from build123d import *

# Parameters (mm, degrees)
BOSS_EXTRUDE1_DEPTH = 3.175
SKETCH2_R           = 1.5875
SKETCH2_W           = 80.264
SKETCH2_H           = 12.954
CUT_EXTRUDE1_DEPTH  = 223.985606318
SKETCH7_R           = 1.5875
SKETCH7_W           = 46.99
SKETCH7_H           = 138.43
CUT_EXTRUDE4_DEPTH  = 223.985606318
CUT_EXTRUDE5_DEPTH  = 223.985606318
SKETCH9_W           = 300.072277348
SKETCH9_H           = 334.026066528
CUT_EXTRUDE6_DEPTH  = 221.482742149
SKETCH10_R          = 1.5875
CUT_EXTRUDE7_DEPTH  = 214.733203623


with BuildPart() as part:
    # Sketch1 → Boss-Extrude1 (new body)
    with BuildSketch(Plane(origin=(0, 0, 0), x_dir=(1, 0, 0), z_dir=(0, 1, 0))):
        with BuildLine():
            Line((-80, 112.5), (100, 112.5))
            Line((100, 112.5), (100, -112.5))
            Line((100, -112.5), (-80, -112.5))
            ThreePointArc((-80, -112.5), (-192.5, 0), (-80, 112.5))
        make_face()
    extrude(amount=-BOSS_EXTRUDE1_DEPTH)

    # Sketch2 → Cut-Extrude1 (cut, through all)
    with BuildSketch(Plane(origin=(0, 0, 0), x_dir=(1, 0, 0), z_dir=(0, 1, 0))):
        with Locations(Location((36.144045702, -74.2188, 0), (0, 0, 270))):
            Circle(SKETCH2_R)
        with Locations(Location((36.144045702, -67.8688, 0), (0, 0, 270))):
            Circle(SKETCH2_R)
        with Locations(Location((36.144045702, -61.5188, 0), (0, 0, 270))):
            Circle(SKETCH2_R)
        with Locations(Location((36.144045702, -55.1688, 0), (0, 0, 270))):
            Circle(SKETCH2_R)
        with Locations(Location((36.144045702, -48.8188, 0), (0, 0, 270))):
            Circle(SKETCH2_R)
        with Locations(Location((36.144045702, -42.4688, 0), (0, 0, 270))):
            Circle(SKETCH2_R)
        with Locations(Location((36.144045702, -36.1188, 0), (0, 0, 270))):
            Circle(SKETCH2_R)
        with Locations(Location((67.894045702, -74.2188, 0), (0, 0, 270))):
            Circle(SKETCH2_R)
        with Locations(Location((67.894045702, -67.8688, 0), (0, 0, 270))):
            Circle(SKETCH2_R)
        with Locations(Location((67.894045702, -61.5188, 0), (0, 0, 270))):
            Circle(SKETCH2_R)
        with Locations(Location((67.894045702, -55.1688, 0), (0, 0, 270))):
            Circle(SKETCH2_R)
        with Locations(Location((67.894045702, -48.8188, 0), (0, 0, 270))):
            Circle(SKETCH2_R)
        with Locations(Location((67.894045702, -42.4688, 0), (0, 0, 270))):
            Circle(SKETCH2_R)
        with Locations(Location((67.894045702, -36.1188, 0), (0, 0, 270))):
            Circle(SKETCH2_R)
        with Locations(Location((36.144045702, 74.2188, 0), (0, 0, 270))):
            Circle(SKETCH2_R)
        with Locations(Location((36.144045702, 67.8688, 0), (0, 0, 270))):
            Circle(SKETCH2_R)
        with Locations(Location((36.144045702, 61.5188, 0), (0, 0, 270))):
            Circle(SKETCH2_R)
        with Locations(Location((36.144045702, 55.1688, 0), (0, 0, 270))):
            Circle(SKETCH2_R)
        with Locations(Location((36.144045702, 48.8188, 0), (0, 0, 270))):
            Circle(SKETCH2_R)
        with Locations(Location((36.144045702, 42.4688, 0), (0, 0, 270))):
            Circle(SKETCH2_R)
        with Locations(Location((36.144045702, 36.1188, 0), (0, 0, 270))):
            Circle(SKETCH2_R)
        with Locations(Location((67.894045702, 74.2188, 0), (0, 0, 270))):
            Circle(SKETCH2_R)
        with Locations(Location((67.894045702, 67.8688, 0), (0, 0, 270))):
            Circle(SKETCH2_R)
        with Locations(Location((67.894045702, 61.5188, 0), (0, 0, 270))):
            Circle(SKETCH2_R)
        with Locations(Location((67.894045702, 55.1688, 0), (0, 0, 270))):
            Circle(SKETCH2_R)
        with Locations(Location((67.894045702, 48.8188, 0), (0, 0, 270))):
            Circle(SKETCH2_R)
        with Locations(Location((67.894045702, 42.4688, 0), (0, 0, 270))):
            Circle(SKETCH2_R)
        with Locations(Location((67.894045702, 36.1188, 0), (0, 0, 270))):
            Circle(SKETCH2_R)
        with Locations((52.019045702, -96.4438)):
            Rectangle(SKETCH2_W, SKETCH2_H)
        with Locations((52.019045702, 96.4438)):
            Rectangle(SKETCH2_W, SKETCH2_H)
    extrude(amount=-CUT_EXTRUDE1_DEPTH, mode=Mode.SUBTRACT)

    # Sketch7 → Cut-Extrude4 (cut, through all)
    with BuildSketch(Plane(origin=(0, 0, 0), x_dir=(1, 0, 0), z_dir=(0, 1, 0))):
        with Locations(Location((-50.166143469, 0, 0), (0, 0, 270))):
            Circle(SKETCH7_R)
        with Locations(Location((25.582761582, 0, 0), (0, 0, 270))):
            Circle(SKETCH7_R)
        with Locations(Location((87.462148806, 0, 0), (0, 0, 270))):
            Circle(SKETCH7_R)
        with Locations((-13.971143469, 0)):
            Rectangle(SKETCH7_W, SKETCH7_H)
    extrude(amount=-CUT_EXTRUDE4_DEPTH, mode=Mode.SUBTRACT)

    # Sketch8 → Cut-Extrude5 (cut, through all)
    with BuildSketch(Plane(origin=(0, 0, 0), x_dir=(1, 0, 0), z_dir=(0, 1, 0))):
        with BuildLine():
            Line((-167.0966, 25.4), (-229.776686608, 25.4))
            Line((-229.776686608, 25.4), (-229.776686608, -25.4))
            Line((-229.776686608, -25.4), (-167.0966, -25.4))
            ThreePointArc((-167.0966, -25.4), (-141.6966, 0), (-167.0966, 25.4))
        make_face()
    extrude(amount=-CUT_EXTRUDE5_DEPTH, mode=Mode.SUBTRACT)

    # Sketch9 → Cut-Extrude6 (cut, through all)
    with BuildSketch(Plane(origin=(0, 0, 0), x_dir=(1, 0, 0), z_dir=(0, 1, 0))):
        with Locations((15.89966987, 0.169857655)):
            Rectangle(SKETCH9_W, SKETCH9_H)
    extrude(amount=-CUT_EXTRUDE6_DEPTH, mode=Mode.SUBTRACT)

    # Sketch10 → Cut-Extrude7 (cut, through all)
    with BuildSketch(Plane(origin=(0, 0, 0), x_dir=(1, 0, 0), z_dir=(0, 1, 0))):
        with Locations(Location((-178.345859252, -36.864745569, 0), (0, 0, 270))):
            Circle(SKETCH10_R)
        with Locations(Location((-178.345859252, 35.885864147, 0), (0, 0, 270))):
            Circle(SKETCH10_R)
    extrude(amount=-CUT_EXTRUDE7_DEPTH, mode=Mode.SUBTRACT)


solid = part.part
Source: CAD feature listing. Evaluate the final solid. Frame: model axes, mm. A direction names the side the tool comes from. Give positions to 0.01 mm unless a question says otherwise; leave off trailing zeros. Write each loop counter-clockwise with the first axis right and the second up, starting at its lowest first coordinate (ties: lowest second). Pieces come first, ordered by that corner, then holes. Notation, with made-up numbers: M 2.5,6.25 L 32.5,6.25 A23 cw 32.5,33.25 Z; hole C 26,46.25 d10. An arc over 180 degrees is marked long. Return JSON: item names as keys, results as strings. Group by question number.
1) Set-up query: faces 5 (the face through (-179, -2, 25.4)), 6 (the face through (-137, 0, -1)). Return all of +Z, -Z, +X, -X, +Y, -Y with unobstructed straight access to the full face (end or side cutting, diameter ignored); none if empty.
2) Cut plane D-D, the plane x = -147. Output: boundary loops of the cut face in (y, z) (3 decimals).
3) Cut plane B-B, the plane y = -1. Output: boundary loops of the cut face in (x, z) (1 decimal).
4) Cut plane C-C, the plane z = 0. Output: boundary loops of the cut face in (x, y) (3 decimals), then the cut area to 3 significant figures.
5) First-contact query: pin 1 Ø10 at (x, z) = (-175.5, -72.5) entering from +Y; pin 2 Ø1.5 at (x, y) = (-142, -2.5) entering from -Z; pin 3 Ø5 at (x, z) = (-178.35, -35.89) entering from +Y; pin 4 Ø1.5 at (x, y) = (-166.5, -2) entering from +Z. Flat tips, straight axial feed; report the tip coordinate or a pass-through.
6) Ray query, L1, parallel to Z at x = -179.5, y = -2.8; L2, parallel to Z at x = -157, y = -2.95; L3, parallel to Z at x = -154, y = -2.2. Return the intervals inside material, ascending.
7) Cut plane A-A, the plane x = -183. Output: boundary loops of the cut face in (y, z) (3 decimals).
8) Draft query along X for faces 1 (the face through (-178, -2, -25.4)), 2 (the face through (-179.9, -1.6, -36.2)), 3 (the face through (-179.896, -1.565, 36.521)), 4 (the face through (-134.136, -2, 1)). Return one class per face: released by +X, released by -X, zero draft, split by the parting line, or undercut.
Data:
{
 "1": {"face 5": "-X, +Y, -Y", "face 6": "+Z, -Z, +X, -X, +Y"},
 "2": {"outline": "M -3.175,-90.373 L 0,-90.373 L 0,-15.533 L -3.175,-15.533 Z; M -3.175,15.533 L 0,15.533 L 0,90.373 L -3.175,90.373 Z"},
 "3": {"outline": "M -189.6,-25.4 A112.5 ccw -134.1,-98.6 L -134.1,98.6 A112.5 ccw -189.6,25.4 L -167.1,25.4 A25.4 cw -167.1,-25.4 Z; hole C -178.3,-35.9 d3.2; hole C -178.3,36.9 d3.2"},
 "4": {"outline": "M -141.697,-3.175 L -134.136,-3.175 L -134.136,0 L -141.697,0 Z", "area": "24.0 mm²"},
 "5": {"pin 1": "passes through", "pin 2": "stops at z = -94.36", "pin 3": "stops at y = 0", "pin 4": "stops at z = 72.82"},
 "6": {"L1": "z = -52.5 to -36.98, -34.8 to -25.4, 25.4 to 35.77, 37.95 to 52.5", "L2": "z = -82.02 to -23.31, 23.31 to 82.02", "L3": "z = -84.74 to -21.76, 21.76 to 84.74"},
 "7": {"outline": "M -3.175,-45.247 L 0,-45.247 L 0,-25.4 L -3.175,-25.4 Z; M -3.175,25.4 L 0,25.4 L 0,45.247 L -3.175,45.247 Z"},
 "8": {"face 1": "zero draft", "face 2": "undercut", "face 3": "undercut", "face 4": "released by +X"}
}
